Geometry: see drawing. Coordinates: mm, zero at the bounding-box minimum. A direction names the side the tool comes from. Coordinates: 2 decimals unless noted, no trailing zeros. Loops run counter-clockwise (first coordinate to the right, second up) from the corner with the lowest first, then second, coordinate; pieces in that order, holes last. Notation, with made-up numbers: (27.25, 39.25) -> (54.25, 39.25) arc R16 ccw to (54.25, 59.25) -> close; hole circle Ø6 at (80, 65.25). An arc over 180 degrees is marked (long way). Answer as a JSON object with one key per item and string values.
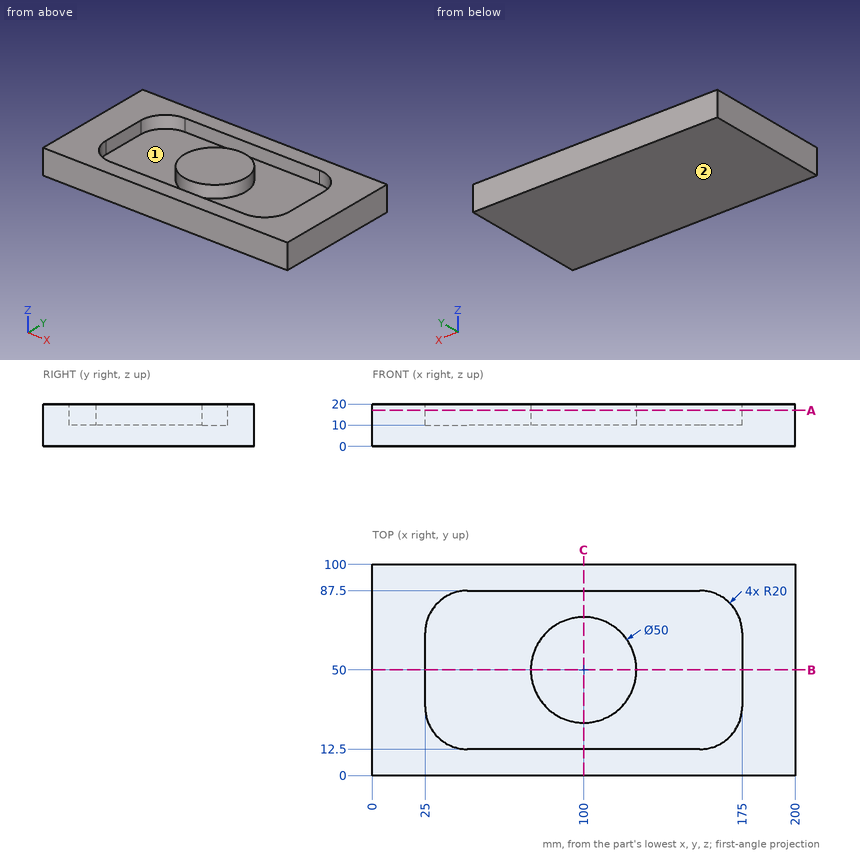
1. Section query A-A (z = 17). Return loops of the section in (x, y).
Reply:
{"outline": "(0, 0) -> (200, 0) -> (200, 100) -> (0, 100) -> close; circle Ø50 at (100, 50); hole (25, 32.5) arc R20 ccw to (45, 12.5) -> (155, 12.5) arc R20 ccw to (175, 32.5) -> (175, 67.5) arc R20 ccw to (155, 87.5) -> (45, 87.5) arc R20 ccw to (25, 67.5) -> close"}
2. Access query for the marked faces 1 and 2. Directions: +Z, -Z, +X, -X, +Y, -Y. A direction counts if a zero-diameter tool reaches every point of the face in a straight line with its end or side. Return the directions, or none.
Reply:
{"face 1": "+Z", "face 2": "-Z, +X, -X, +Y, -Y"}
3. Line query: line 1 along Y through (x, z) = (112, 14.25); line 2 along Y through (x, z) = (84.5, 15.5); line 3 along Y through (x, z) = (47.5, 13.5). Output: solid intervals per line, ascending.
Reply:
{"line 1": "y = 0 to 12.5, 28.07 to 71.93, 87.5 to 100", "line 2": "y = 0 to 12.5, 30.38 to 69.62, 87.5 to 100", "line 3": "y = 0 to 12.5, 87.5 to 100"}
4. Section query B-B (y = 50). Return loops of the section in (x, z).
Reply:
{"outline": "(0, 0) -> (200, 0) -> (200, 20) -> (175, 20) -> (175, 10) -> (125, 10) -> (125, 20) -> (75, 20) -> (75, 10) -> (25, 10) -> (25, 20) -> (0, 20) -> close"}
5. Section query C-C (x = 100). Return loops of the section in (y, z).
Reply:
{"outline": "(0, 0) -> (100, 0) -> (100, 20) -> (87.5, 20) -> (87.5, 10) -> (75, 10) -> (75, 20) -> (25, 20) -> (25, 10) -> (12.5, 10) -> (12.5, 20) -> (0, 20) -> close"}
6. Pin query (flat end, axial travel): P1, Ø8, axis at x = 136.5, y = 32.5, coming from the +Z side; P2, Ø8, axis at y = 63, z = 4, coming from the -X side. Return the tip coordinate at first contact, or that it passes through.
Reply:
{"P1": "stops at z = 10", "P2": "stops at x = 0"}
